Check sheet for the modelled part. Datum: model origin and axes. Units: mm. Give positions to 0.01 mm unless a question says otherwise; leave off trailing zeros. Loops run counter-clockwise (first coordinate to the right, second up) from the corner with the lowest first, then second, coordinate; pieces in that order, holes last. Notation, with made-up numbers: M 3.25,16.25 L 31.25,16.25 A22 ccw 31.25,27.25 Z; hole C -5.5,-26 d2. An arc over 180 degrees is marked long. Put each result on its own line as item: value. Start each with the question number.
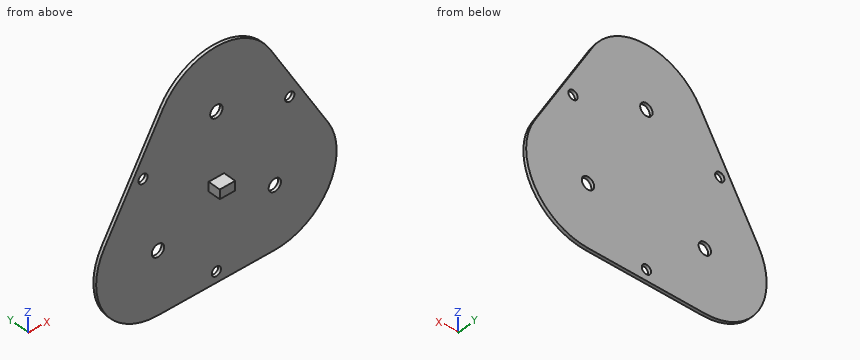
```python
from build123d import *

# Parameters (mm, degrees)
SKETCH1_R           = 2
SKETCH1_R_2         = 1.5
BOSS_EXTRUDE1_DEPTH = 1
SKETCH2_W           = 5
SKETCH2_H           = 3
BOSS_EXTRUDE2_DEPTH = 4


with BuildPart() as part:
    # Sketch1 → Boss-Extrude1 (new body)
    with BuildSketch(Plane(origin=(0, 0, 0), x_dir=(1, 0, 0), z_dir=(0, 1, 0))):
        with BuildLine():
            Line((36.224008076, 0.913940814), (17.320508076, -31.827881627))
            ThreePointArc((17.320508076, -31.827881627), (0, -41.827881627), (-17.320508076, -31.827881627))
            Line((-17.320508076, -31.827881627), (-36.224008076, 0.913940814))
            ThreePointArc((-36.224008076, 0.913940814), (-36.224008076, 20.913940814), (-18.9035, 30.913940814))
            Line((-18.9035, 30.913940814), (18.9035, 30.913940814))
            ThreePointArc((18.9035, 30.913940814), (36.224008076, 20.913940814), (36.224008076, 0.913940814))
        make_face()
        with Locations((-18.9035, 10.913940814)):
            Circle(SKETCH1_R, mode=Mode.SUBTRACT)
        with Locations((18.9035, 10.913940814)):
            Circle(SKETCH1_R, mode=Mode.SUBTRACT)
        with Locations((0, -21.827881627)):
            Circle(SKETCH1_R, mode=Mode.SUBTRACT)
        with Locations((-23.741169162, -13.706970407)):
            Circle(SKETCH1_R_2, mode=Mode.SUBTRACT)
        with Locations((23.741169162, -13.706970407)):
            Circle(SKETCH1_R_2, mode=Mode.SUBTRACT)
        with Locations((0, 27.413940814)):
            Circle(SKETCH1_R_2, mode=Mode.SUBTRACT)
    extrude(amount=BOSS_EXTRUDE1_DEPTH)

    # Sketch2 → Boss-Extrude2 (add)
    with BuildSketch(Plane.XZ):
        Rectangle(SKETCH2_W, SKETCH2_H)
    extrude(amount=BOSS_EXTRUDE2_DEPTH)


solid = part.part
```
Q1. Depth check by flat-ended pin: P1, Ø5, axis at x = 9, z = 18.5, coming from the -Y side; P2, Ø1.2, axis at x = 0, y = -2.5, coming from the +Z side; P3, Ø2.5, axis at x = -23.74, z = 13.71, coming from the -Y side; P4, Ø2, axis at x = 1, y = -1.5, coming from the -Z side. Enter the tip coordinate at first touch or a pass-through.
Q2. Section check C-C, the plane x = -28.5. Record the cut outline in (y, z), then the cut area to 3 significant figures.
Q3. Section check A-A, the plane x = 0. Record the cut outline in (y, z), then the cut area to 3 significant figures.
Q4. Section check B-B, the plane y = -2.7. Record the cut outline in (x, z).
Q5. Thickness scan on line 1 along Z through (x, y) = (0, 0.4); line 2 along Y through (x, z) = (-5, -13.5); line 3 along Z through (x, y) = (-1, -0.65). Record the ranges inside material, lowest first. Write a range as [from, to].
Found:
1. P1: stops at y = 0
1. P2: stops at z = 1.5
1. P3: passes through
1. P4: stops at z = -1.5
2. outline: M 0,-28.46 L 1,-28.46 L 1,12.46 L 0,12.46 Z
2. area: 40.9 mm^2
3. outline: M -4,-1.5 L 0,-1.5 L 0,-25.91 L 1,-25.91 L 1,19.83 L 0,19.83 L 0,1.5 L -4,1.5 Z; M 0,-30.91 L 1,-30.91 L 1,-28.91 L 0,-28.91 Z; M 0,23.83 L 1,23.83 L 1,41.83 L 0,41.83 Z
3. area: 77.7 mm^2
4. outline: M -2.5,-1.5 L 2.5,-1.5 L 2.5,1.5 L -2.5,1.5 Z
5. line 1: z = [-30.91, -28.91], [-25.91, 19.83], [23.83, 41.83]
5. line 2: y = [0, 1]
5. line 3: z = [-1.5, 1.5]
